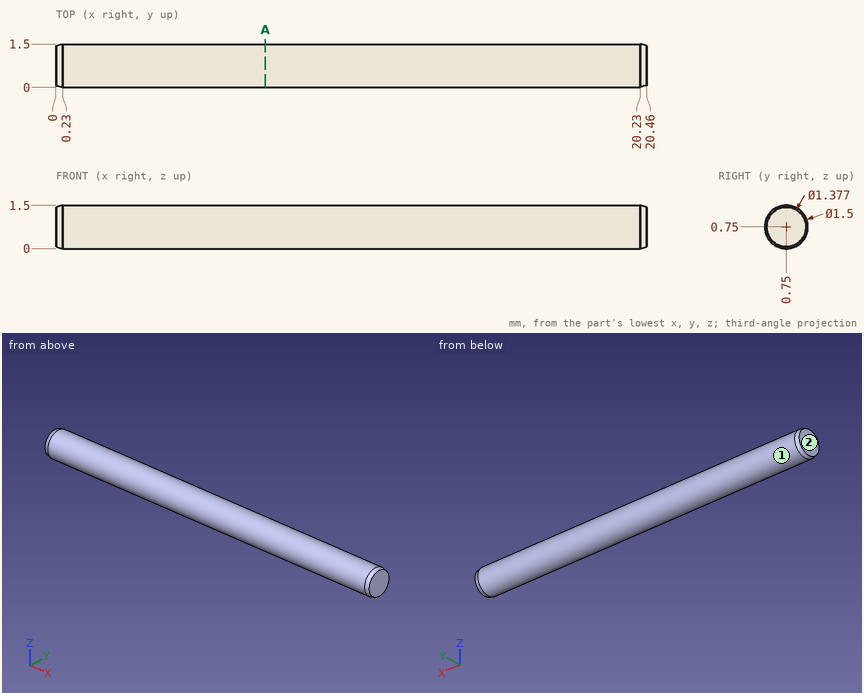
Job drawing, mm, ordinate dimensions from the low corner. One solid piece. Coordinates: 2 decimals unless noted, no trailing zeros. Order: outer loops, then holes, each group sorted by start corner. A loop starts at its lowest first (then second) coordinate and runs counter-clockwise, first axis right, second up. Notation, with made-up numbers: M -22.5,-1.5 L 19.5,-1.5 A24 cw 19.5,33.5 Z; hole C -2.75,42.25 d4. An arc over 180 degrees is marked long. Answer as CSV lines item,"result".
(1) Pull direction Z, two halves, no side cores. Call the marked faces 1 and 2: +Z half, -Z half, draft (parallel to the pull), parting line (faces both ways), or undercut.
Geometry says:
face 1,"parting line"
face 2,"draft"
(2) Wall check: line 1 along Z through (x, y) = (15.5, 0.7); line 2 along Z through (x, y) = (5.75, 1.1). Give the ranges that are in metal, low to high.
Geometry says:
line 1,"z = 0 to 1.5"
line 2,"z = 0.09 to 1.41"
(3) Band-saw the part on A-A, the plane x = 7.25. List the corners of the cut face in (y, z).
Geometry says:
outline,"C 0.75,0.75 d1.5"
